Answer from the drawing. Dimensions are ordinates in mm from the lowest x, y and z of the part. Give positions to 0.01 mm unless a question says otherwise; leave off trailing zeros. Write each loop counter-clockwise with the first axis right and the second up, starting at its lowest first coordinate (ties: lowest second). Pieces come first, ordered by that corner, then holes. Notation, with made-up numbers: (22.25, -30) -> (79.25, -30) arc R21 ccw to (79.25, -9) -> close; hole circle Ø8 at (-24.75, 30). An arc over 180 degrees is marked (long way). Use a Markdown table: item, result. Add a question column.
Q1. Section B-B, the plane x = 12.7 is taken. Give the vertices of the cut face in (y, z), plus the area to 3 significant figures.
Q2. Section A-A, the plane z = 12.7 is taken. Give the vertices of the cut face in (x, y), plus the area to 3 significant figures.
Q3. Consider line 1 (X direction, y = 5.1, z = 12.7); line 2 (X direction, y = 4, z = 11.5) (1 decimal); line 3 (Z direction, x = 12.7, y = 4.8). Determine where each line is inside the solid, lowest interval first.
Q4. Section C-C, the plane y = 4.75 is taken. Give the vertices of the cut face in (x, z), plus the area to 3 significant figures.
Q5. Each of these flat-tipped pins is pushed along its axis until it touches: pin 1 Ø10.5 at (x, z) = (12.7, 12.7) entering from -Y; pin 2 Ø1.5 at (x, z) = (225, 3.5) entering from -Y; pin 3 Ø7.5 at (x, z) = (241.3, 12.7) entering from -Y (1 decimal). Where does it stop, or does it pass through?
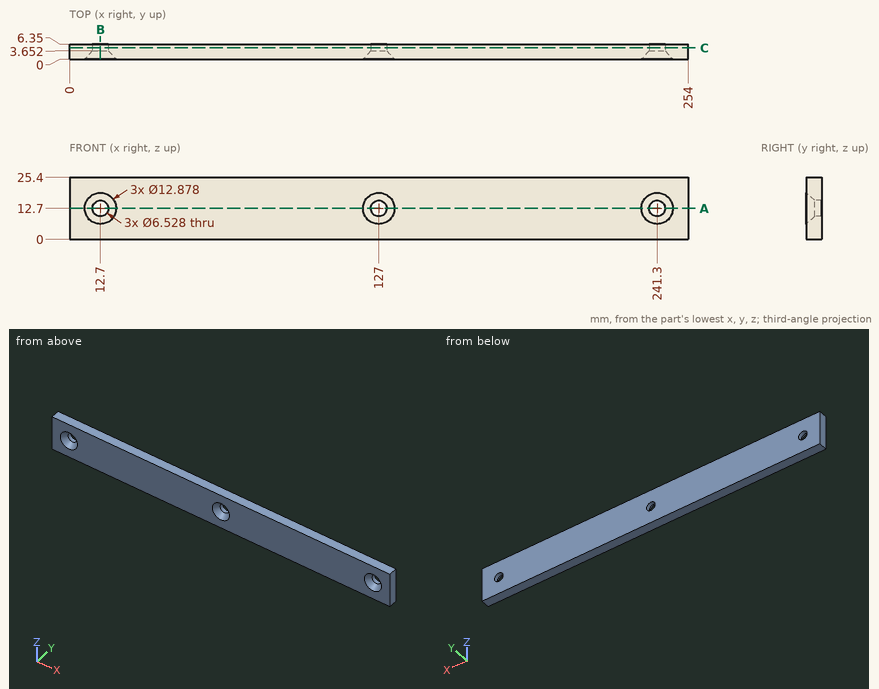
Result set:
| question | item | result |
|---|---|---|
| 1 | outline | (0, 0) -> (6.35, 0) -> (6.35, 9.44) -> (3.65, 9.44) -> (0, 6.26) -> close; (0, 19.14) -> (3.65, 15.96) -> (6.35, 15.96) -> (6.35, 25.4) -> (0, 25.4) -> close |
| 1 | area | 108 mm2 |
| 2 | outline | (0, 0) -> (6.26, 0) -> (9.44, 3.65) -> (9.44, 6.35) -> (0, 6.35) -> close; (15.96, 3.65) -> (19.14, 0) -> (120.56, 0) -> (123.74, 3.65) -> (123.74, 6.35) -> (15.96, 6.35) -> close; (130.26, 3.65) -> (133.44, 0) -> (234.86, 0) -> (238.04, 3.65) -> (238.04, 6.35) -> (130.26, 6.35) -> close; (244.56, 3.65) -> (247.74, 0) -> (254, 0) -> (254, 6.35) -> (244.56, 6.35) -> close |
| 2 | area | 1,450 mm2 |
| 3 | line 1 | x = 0 to 9.44, 15.96 to 123.74, 130.26 to 238.04, 244.56 to 254 |
| 3 | line 2 | x = 0 to 9.7, 15.7 to 124, 130 to 238.3, 244.3 to 254 |
| 3 | line 3 | z = 0 to 9.44, 15.96 to 25.4 |
| 4 | outline | (0, 0) -> (254, 0) -> (254, 25.4) -> (0, 25.4) -> close; hole circle Ø6.53 at (12.7, 12.7); hole circle Ø6.53 at (127, 12.7); hole circle Ø6.53 at (241.3, 12.7) |
| 4 | area | 6,350 mm2 |
| 5 | pin 1 | stops at y = 1.37 |
| 5 | pin 2 | stops at y = 0 |
| 5 | pin 3 | stops at y = 3.1 |
